```python
from build123d import *

# Parameters (mm, degrees)
F0_W     = 76.2
F0_H     = 50.8
F1_DEPTH = 38.1
F4_W     = 76.2
F4_H     = 50.8
F4_W_2   = 74.2
F4_H_2   = 48.8
F5_DEPTH = 1
F2_R     = 1.5875
F6_DEPTH = 25.4


with BuildPart() as f1:
    # F0 (on Top) → F1 (new body)
    with BuildSketch(Plane.XY):
        Rectangle(F0_W, F0_H)
    extrude(amount=F1_DEPTH)

    # F4 (on offset) → F5 (cut)
    with BuildSketch(Plane.XY.offset(25.4)):
        Rectangle(F4_W, F4_H)
        Rectangle(F4_W_2, F4_H_2, mode=Mode.SUBTRACT)
    extrude(amount=F5_DEPTH, mode=Mode.SUBTRACT)

    # F2 (on face) → F6 (cut)
    with BuildSketch(Plane(origin=(-38.1, 0, 0), x_dir=(0, -1, 0), z_dir=(-1, 0, 0))):
        with Locations((-12.7, 19.05)):
            Circle(F2_R)
        with Locations((12.7, 19.05)):
            Circle(F2_R)
    extrude(amount=-F6_DEPTH, mode=Mode.SUBTRACT)


solid = f1.part
```
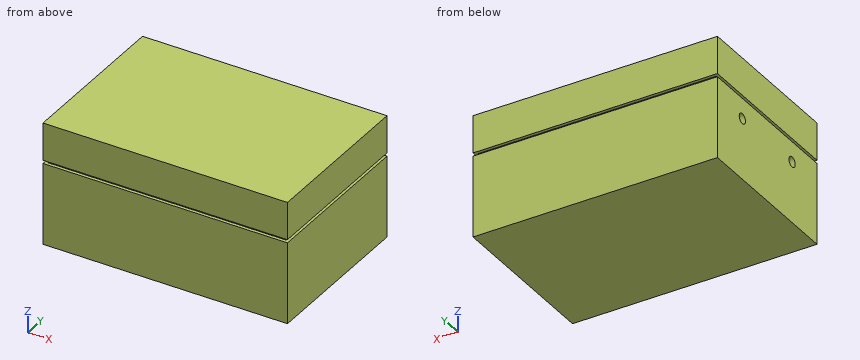
Design review of the part built by this model. Coordinates are the model's own, in mm. Coordinates: 2 decimals unless noted, no trailing zeros. Write each loop counter-clockwise with the first axis right and the second up, starting at its lowest first coordinate (ties: lowest second). Pieces come first, ordered by that corner, then holes.
1) Add section A-A (z = 19.05). Write out the cut boundary in (x, y).
2) To check wall thickness, follow L1, parallel to Y at x = -22, z = 19; L2, parallel to Z at x = -21, y = 12.7; L3, parallel to Z at x = -21, y = 12. State the ranges of each line that lie inside material, in increasing order.
3) Add section B-B (y = -12.7). Write out the cut boundary in (x, z), plus the area to 3 significant figures.
4) Insertion check: pin 1 (1.1 mm diameter, centred on y = 1, z = 26, fed in from +X); pin 2 (0.5 mm diameter, centred on x = -5, z = 26, fed in from +Y). Each pin has a flat end and moves straight along its axis. Give the tip position at first contact, or say it passes through.
5) Add section C-C (y = 12). Write out the cut boundary in (x, z).
Check result:
1. outline: (-38.1, -25.4) - (38.1, -25.4) - (38.1, 25.4) - (-38.1, 25.4) - (-38.1, 14.29) - (-12.7, 14.29) - (-12.7, 11.11) - (-38.1, 11.11) - (-38.1, -11.11) - (-12.7, -11.11) - (-12.7, -14.29) - (-38.1, -14.29) - close
2. L1: y = -25.4 to -14.29, -11.11 to 11.11, 14.29 to 25.4
2. L2: z = 0 to 17.46, 20.64 to 38.1
2. L3: z = 0 to 17.63, 20.47 to 38.1
3. outline: (-38.1, 0) - (38.1, 0) - (38.1, 25.4) - (37.1, 25.4) - (37.1, 26.4) - (38.1, 26.4) - (38.1, 38.1) - (-38.1, 38.1) - (-38.1, 26.4) - (-37.1, 26.4) - (-37.1, 25.4) - (-38.1, 25.4) - (-38.1, 20.64) - (-12.7, 20.64) - (-12.7, 17.46) - (-38.1, 17.46) - close
3. area: 2,820 mm2
4. pin 1: stops at x = 38.1
4. pin 2: stops at y = 24.4
5. outline: (-38.1, 0) - (38.1, 0) - (38.1, 25.4) - (37.1, 25.4) - (37.1, 26.4) - (38.1, 26.4) - (38.1, 38.1) - (-38.1, 38.1) - (-38.1, 26.4) - (-37.1, 26.4) - (-37.1, 25.4) - (-38.1, 25.4) - (-38.1, 20.47) - (-12.7, 20.47) - (-12.7, 17.63) - (-38.1, 17.63) - close
